Autodesk Inventor part; units mm, degrees
ref_plane "YZ Plane" through (0, 0, 0) normal (1, 0, 0) x (0, 1, 0)
ref_plane "XZ Plane" through (0, 0, 0) normal (0, 1, 0) x (-1, 0, 0)
ref_plane "XY Plane" through (0, 0, 0) normal (0, 0, 1) x (1, 0, 0)
sketch "Sketch1" plane through (0, 0, 0) normal (1, 0, 0) x (0, 1, 0)
  line L0 (-76.2, 88.9) -> (-76.2, 88.9)
  line L1 (-50.8, 127) -> (50.8, 127)
  line L2 (50.8, -127) -> (-50.8, -127)
  line L3 (-76.2, -88.9) -> (-76.2, 88.9)
  arc A0 (88.9, 88.9) -> (50.8, 127) centre (50.8, 88.9) ccw
  line L4 (76.2, 88.9) -> (88.9, 88.9)
  arc A1 (-50.8, 127) -> (-88.9, 88.9) centre (-50.8, 88.9) ccw
  line L5 (-50.8, 88.9) -> (-88.9, 88.9)
  arc A2 (50.8, -127) -> (88.9, -88.9) centre (50.8, -88.9) ccw
  line L6 (76.2, -88.9) -> (88.9, -88.9)
  line L7 (76.2, 88.9) -> (76.2, -88.9)
  arc A3 (-88.9, -88.9) -> (-50.8, -127) centre (-50.8, -88.9) ccw
  line L8 (-76.2, -88.9) -> (-88.9, -88.9)
  point P0 (0, 0)
  point P1 (-76.2, 117.2981)
  point P2 (-76.2, -117.2981)
  dimension "d62" = 254
  dimension "d64" = 76.2
  dimension "d65" = 127
  dimension "d66" = 76.2
  dimension "d72" = 76.2
  dimension "d73" = 25.4
  dimension "d74" = 76.2
  dimension "d76" = 25.4
  dimension "d77" = 76.2
  dimension "d78" = 25.4
extrude "Extrusion1" add sketch "Sketch1" along normal blind 5.08
sketch "Sketch3" plane through (5.08, 0, 0) normal (1, 0, 0) x (0, 0, -1)
  line L0 (88.9, 76.2) -> (-88.9, 76.2)
  line L1 (127, -50.8) -> (127, 50.8)
  line L2 (-88.9, -76.2) -> (88.9, -76.2)
  point P0 (0, 0)
  point P1 (0, -63.5)
  point P2 (0, 63.5)
  point P3 (0, 63.5)
  point P4 (127, 76.2)
  point P5 (127, -76.2)
  point P6 (-127, -76.2)
  dimension "d68" = 12.7
  dimension "d69" = 127
  dimension "d70" = 127
  dimension "d71" = 12.7
hole "Hole2" at (5.08, -63.5, 0) direction (-1, 0, 0) diameter 6.35 end through all
hole "Hole3" at (5.08, 63.5, 0) direction (-1, 0, 0) diameter 6.35 end through all
sketch "Sketch4" plane through (5.08, 0, 0) normal (1, 0, 0) x (0, 0, -1)
  line L0 (-127, 50.8) -> (-127, -50.8)
  line L1 (-127, 50.8) -> (127, 50.8)
  line L2 (127, 50.8) -> (127, -50.8)
  line L3 (127, -50.8) -> (-127, -50.8)
  line L4 (-127, -50.8) -> (-127, 50.8)
  point P0 (0, 0)
  point P1 (-88.9, 88.9)
  dimension "d79" = 101.6
  dimension "d80" = 38.1
extrude "Extrusion2" add sketch "Sketch4" against normal blind 8.255
properties part number "Frame 2.0" material "ABS Plastic"
Here's how the part is built. I have some questions about the finished solid (model axes, mm). A direction names the side the tool comes from. Round coordinates to 2 decimals unless told otherwise and drop trailing zeros. Loops run counter-clockwise (first coordinate to the right, second up) from the corner with the lowest first, then second, coordinate; pieces in that order, holes last. Notation, with made-up numbers: (49.5, 56) - (54.5, 56) arc R15 ccw to (54.5, 80) - close; hole circle Ø9 at (9.5, 81). An arc over 180 degrees is marked (long way). One line per question, with ' | ' between items. Start each with the question number.
Q1. We'd pull the mould along Z, two halves only. Please class faces 5 (the cylindrical face through (2.504, -66.177, -1.707)), 6 (the cylindrical face through (2.5, -77.44, -116.14)), 7 (the cylindrical face through (2.5, -78.04, 115.54)): +Z half, -Z half, draft (parallel to the pull), parting line (faces both ways), or undercut.
Q2. I want a section at D-D (z = -78). Write out the boundary of the cut face in (x, y) (3 decimals), then the cut area to 3 significant figures.
Q3. Will these pins go through, and if not, where does the flat tip stop? pin 1 (11.5 mm diameter, centred on y = -67, z = -39, fed in from -X); pin 2 (1.5 mm diameter, centred on x = 2.5, z = 41, fed in from -Y); pin 3 (2.5 mm diameter, centred on x = 3, y = -83.5, fed in from -Z); pin 4 (10 mm diameter, centred on y = 63.5, z = 0, fed in from +X).
Q4. I want a section at B-B (x = 2.5). Write out the boundary of the cut face in (y, z) (3 decimals).
Q5. I want a section at C-C (y = -63.5). Write out the boundary of the cut face in (x, z) (3 decimals), then the cut area to 3 significant figures.
Q6. For faces 1 (the flat face through (3, 76.2, 1)), 2 (the flat face through (0, 70, 2)), 3 (the flat face through (3, -76.2, -1)), 4 (the flat face through (0, -70, 2)), which set-ups out of +Z, -Z, +X, -X, +Y, -Y let a thin tool reach every point of the face, with its end or its side?
Q7. Please list where these lines run through material, in increasing order: line 1 (Y direction, x = 3.35, z = 0) (3 decimals); line 2 (Y direction, x = 1.75, z = -38); line 3 (X direction, y = -63.5, z = 69). Write a range as [from, to].
Q8. I want a section at A-A (z = 0). Write out the boundary of the cut face in (x, y) (3 decimals), then the cut area to 3 significant figures.
Response values:
1) face 5: undercut | face 6: -Z half | face 7: +Z half
2) outline: (-3.175, -50.8) - (0, -50.8) - (0, -76.2) - (5.08, -76.2) - (5.08, 76.2) - (0, 76.2) - (0, 50.8) - (-3.175, 50.8) - close | area: 1,100 mm²
3) pin 1: stops at x = 0 | pin 2: stops at y = -76.2 | pin 3: stops at z = -110.41 | pin 4: stops at x = 5.08
4) outline: (-88.9, -88.9) arc R38.1 ccw to (-50.8, -127) - (50.8, -127) arc R38.1 ccw to (88.9, -88.9) - (76.2, -88.9) - (76.2, 88.9) - (88.9, 88.9) arc R38.1 ccw to (50.8, 127) - (-50.8, 127) arc R38.1 ccw to (-88.9, 88.9) - (-76.2, 88.9) - (-76.2, -88.9) - close; hole circle Ø6.35 at (-63.5, 0); hole circle Ø6.35 at (63.5, 0)
5) outline: (0, -124.821) - (5.08, -124.821) - (5.08, -3.175) - (0, -3.175) - close; (0, 3.175) - (5.08, 3.175) - (5.08, 124.821) - (0, 124.821) - close | area: 1,240 mm²
6) face 1: +X, -X, +Y | face 2: +Z, -Z, -X, +Y | face 3: +X, -X, -Y | face 4: +Z, -Z, -X, -Y
7) line 1: y = [-76.2, -66.675], [-60.325, 60.325], [66.675, 76.2] | line 2: y = [-76.2, 76.2] | line 3: x = [0, 5.08]
8) outline: (-3.175, -50.8) - (0, -50.8) - (0, -60.325) - (5.08, -60.325) - (5.08, 60.325) - (0, 60.325) - (0, 50.8) - (-3.175, 50.8) - close; (0, -76.2) - (5.08, -76.2) - (5.08, -66.675) - (0, -66.675) - close; (0, 66.675) - (5.08, 66.675) - (5.08, 76.2) - (0, 76.2) - close | area: 1,030 mm²
